Model file for the job. Use its own axes, mm. A direction names the side the tool comes from. Coordinates: 2 decimals unless noted, no trailing zeros. Write each loop counter-clockwise with the first axis right and the second up, starting at its lowest first coordinate (ties: lowest second). Pieces come first, ordered by that corner, then holes.
Q1. Band-saw the part on A-A, the plane x = 0. State how many separate pieces and enclosed holes the cut face has, plus the area to 3 significant figures.
Q2. Which spindle directions (+Z, -Z, +X, -X, +Y, -Y) get a long thin tool onto all of the face, cutting with end or side? Do faces 5 (the cylindrical face through (-0.91, 8.437, -0.626)), 6 (the cylindrical face through (6.09, 1.24, -4.28)), 7 (the flat face through (0, -4, -18.263)). Say none if no direction does.
Q3. Pin check, flat tips, straight feed: P1, Ø3, axis at x = -1.5, y = 2.5, coming from the +Z side; P2, Ø1.9, axis at x = 7.493, z = -20.828, coming from the +Y side. Stop position of each tip, or through.
Q4. Drill centre lines: probe 1 along Z at (x, y) = (6.25, -3); probe 2 along Z at (x, y) = (4, 6.75); probe 3 along X at (y, z) = (1.5, -14.25). Where is each one in solid material? Low to high.
Q5. Pull direction Z, two halves, no side cores. Call faces 1 (the flat face through (0, -2, -18.288)), 2 (the flat face through (0, -4, -17.475)), 3 (the flat face through (3, -4, -7.366)), 4 (the flat face through (1, -8.496, -15)): released by +Z, released by -Z, zero draft, split by the parting line, or undercut.
Q6. Band-saw the part on B-B, the plane y = -7. Write the cut outline in (x, z).
from build123d import *

# Parameters (mm, degrees)
SKETCH1_W           = 14.986
SKETCH1_H           = 16.9926
BOSS_EXTRUDE4_DEPTH = 24.1554
SKETCH10_R          = 1.4224
CUT_EXTRUDE6_DEPTH  = 24.1554
SKETCH11_R          = 3.2639
CUT_EXTRUDE7_DEPTH  = 19.558
SKETCH12_R          = 5.1308
CUT_EXTRUDE8_DEPTH  = 18.288
SKETCH13_W          = 14.986
SKETCH13_H          = 16.9926
SKETCH13_R          = 5.1308
CUT_EXTRUDE9_DEPTH  = 7.366
BOSS_EXTRUDE5_START = 6.096
SKETCH14_R          = 6.096
SKETCH14_R_2        = 5.1308
BOSS_EXTRUDE5_DEPTH = 6.096
BOSS_EXTRUDE6_START = 1.27
SKETCH15_R          = 6.9926
SKETCH15_R_2        = 5.1308
BOSS_EXTRUDE6_DEPTH = 1.27
SKETCH16_W          = 14.986
SKETCH16_H          = 16.9926
CUT_EXTRUDE10_DEPTH = 0.7874
SKETCH18_W          = 16.002
SKETCH18_H          = 16.9926
BOSS_EXTRUDE7_DEPTH = 2.54
SKETCH19_R          = 0.8382
CUT_EXTRUDE11_DEPTH = 20.32
SKETCH24_W          = 13.1826
SKETCH24_H          = 0.7874
CUT_EXTRUDE14_DEPTH = 16.256


with BuildPart() as part:
    # Sketch1 → Boss-Extrude4 (new body)
    with BuildSketch(Plane.XY):
        Rectangle(SKETCH1_W, SKETCH1_H)
    extrude(amount=-BOSS_EXTRUDE4_DEPTH)

    # Sketch10 → Cut-Extrude6 (cut)
    with BuildSketch(Plane.XY):
        with Locations((0, 1.5037)):
            Circle(SKETCH10_R)
    extrude(amount=-CUT_EXTRUDE6_DEPTH, mode=Mode.SUBTRACT)

    # Sketch11 → Cut-Extrude7 (cut)
    with BuildSketch(Plane.XY):
        with Locations((0, 1.5037)):
            Circle(SKETCH11_R)
    extrude(amount=-CUT_EXTRUDE7_DEPTH, mode=Mode.SUBTRACT)

    # Sketch12 → Cut-Extrude8 (cut)
    with BuildSketch(Plane.XY):
        with Locations((0, 1.5037)):
            Circle(SKETCH12_R)
    extrude(amount=-CUT_EXTRUDE8_DEPTH, mode=Mode.SUBTRACT)

    # Sketch13 → Cut-Extrude9 (cut)
    with BuildSketch(Plane.XY):
        Rectangle(SKETCH13_W, SKETCH13_H)
        with Locations((0, 1.5037)):
            Circle(SKETCH13_R, mode=Mode.SUBTRACT)
    extrude(amount=-CUT_EXTRUDE9_DEPTH, mode=Mode.SUBTRACT)

    # Sketch14 → Boss-Extrude5 (add)
    with BuildSketch(Plane.XY.offset(-7.366).offset(BOSS_EXTRUDE5_START)):
        with Locations(Location((0, 1.5037, 0), (0, 0, 180))):
            Circle(SKETCH14_R)
        with Locations((0, 1.5037)):
            Circle(SKETCH14_R_2, mode=Mode.SUBTRACT)
    extrude(amount=-BOSS_EXTRUDE5_DEPTH)

    # Sketch15 → Boss-Extrude6 (add)
    with BuildSketch(Plane.XY.offset(-1.27).offset(BOSS_EXTRUDE6_START)):
        with Locations((0, 1.5037)):
            Circle(SKETCH15_R)
        with Locations((0, 1.5037)):
            Circle(SKETCH15_R_2, mode=Mode.SUBTRACT)
    extrude(amount=-BOSS_EXTRUDE6_DEPTH)

    # Sketch16 → Cut-Extrude10 (cut)
    with BuildSketch(Plane(origin=(0, 0, -24.1554), x_dir=(-1, 0, 0), z_dir=(0, 0, -1))):
        Rectangle(SKETCH16_W, SKETCH16_H)
    extrude(amount=-CUT_EXTRUDE10_DEPTH, mode=Mode.SUBTRACT)

    # Sketch18 → Boss-Extrude7 (add)
    with BuildSketch(Plane(origin=(7.493, 0, 0), x_dir=(0, 0, -1), z_dir=(1, 0, 0))):
        with Locations((15.367, 0)):
            Rectangle(SKETCH18_W, SKETCH18_H)
    extrude(amount=BOSS_EXTRUDE7_DEPTH)

    # Sketch19 → Cut-Extrude11 (cut)
    with BuildSketch(Plane(origin=(0, 8.4963, 0), x_dir=(1, 0, 0), z_dir=(0, 1, 0))):
        with Locations(Location((-4.953, 20.828, 0), (0, 0, 270))):
            Circle(SKETCH19_R)
        with Locations(Location((7.493, 20.828, 0), (0, 0, 270))):
            Circle(SKETCH19_R)
        with Locations(Location((7.493, 9.906, 0), (0, 0, 270))):
            Circle(SKETCH19_R)
    extrude(amount=-CUT_EXTRUDE11_DEPTH, mode=Mode.SUBTRACT)

    # Cut-Extrude13 cone 1 section (through the dimple's axis) → Cut-Extrude13 (revolve, cut)
    with BuildSketch(Plane(origin=(-4.953, 8.4963, -20.828), x_dir=(0, 0, 1), z_dir=(1, 0, 0))):
        Polygon((0, 0), (1.4224, 0), (0, 0.199905283), align=None)
    revolve(axis=Axis((-4.953, 8.4963, -20.828), (0, -1, 0)), mode=Mode.SUBTRACT)

    # Cut-Extrude13 cone 2 section (through the dimple's axis) → Cut-Extrude13 cone 2 (revolve, cut)
    with BuildSketch(Plane(origin=(7.493, 8.4963, -20.828), x_dir=(0, 0, 1), z_dir=(1, 0, 0))):
        Polygon((0, 0), (1.4224, 0), (0, 0.199905283), align=None)
    revolve(axis=Axis((7.493, 8.4963, -20.828), (0, -1, 0)), mode=Mode.SUBTRACT)

    # Cut-Extrude13 cone 3 section (through the dimple's axis) → Cut-Extrude13 cone 3 (revolve, cut)
    with BuildSketch(Plane(origin=(7.493, 8.4963, -9.906), x_dir=(0, 0, 1), z_dir=(1, 0, 0))):
        Polygon((0, 0), (1.4224, 0), (0, 0.199905283), align=None)
    revolve(axis=Axis((7.493, 8.4963, -9.906), (0, -1, 0)), mode=Mode.SUBTRACT)

    # Sketch24 → Cut-Extrude14 (cut)
    with BuildSketch(Plane.XZ.offset(8.4963)):
        with Locations((0, -17.8689)):
            Rectangle(SKETCH24_W, SKETCH24_H)
    extrude(amount=-CUT_EXTRUDE14_DEPTH, mode=Mode.SUBTRACT)


solid = part.part
Answer sheet:
1. separate pieces: 3
1. enclosed holes: 0
1. area: 152 mm2
2. face 5: +Z
2. face 6: none
2. face 7: -Y
3. P1: stops at z = -18.29
3. P2: stops at y = 8.43
4. probe 1: z = -23.37 to -18.26, -17.48 to -7.37
4. probe 2: z = -23.37 to -18.26, -17.48 to -7.37, -1.27 to 0
4. probe 3: x = -7.49 to -5.13, 5.13 to 10.03
5. face 1: released by +Z
5. face 2: undercut
5. face 3: undercut
5. face 4: zero draft
6. outline: (-7.49, -23.37) - (10.03, -23.37) - (10.03, -7.37) - (-7.49, -7.37) - close; hole (-6.59, -18.26) - (6.59, -18.26) - (6.59, -17.48) - (-6.59, -17.48) - close; hole circle Ø1.68 at (-4.95, -20.83); hole circle Ø1.68 at (7.49, -20.83); hole circle Ø1.68 at (7.49, -9.91)
